from build123d import *

# Parameters (mm, degrees)
SKETCH_1_W           = 600
SKETCH_1_H           = 100
EXTRUDE_1_DEPTH      = 20
SKETCH_2_W           = 20
SKETCH_2_H           = 100
EXTRUDE_2_DEPTH      = 74
EXTRUDE_3_DEPTH      = 300
EXTRUDE_3_DEPTH_BACK = 300
SKETCH_3_W           = 20
SKETCH_3_H           = 20


with BuildPart() as part:
    # Эскиз1 → Выдавливание1 (new body)
    with BuildSketch(Plane(origin=(0, 0, 0), x_dir=(-1, 0, 0), z_dir=(0, 1, 0))):
        Rectangle(SKETCH_1_W, SKETCH_1_H)
    extrude(amount=EXTRUDE_1_DEPTH)

    # Эскиз2 → Выдавливание2 (add)
    with BuildSketch(Plane(origin=(0, 20, 0), x_dir=(-1, 0, 0), z_dir=(0, 1, 0))):
        with Locations((-290, 0)):
            Rectangle(SKETCH_2_W, SKETCH_2_H)
        with Locations((290, 0)):
            Rectangle(SKETCH_2_W, SKETCH_2_H)
    extrude(amount=EXTRUDE_2_DEPTH)

    # Эскиз3 → Выдавливание3 (add, two sides: drawn at the far end of the back side and taken through both)
    with BuildSketch(Plane.YZ.offset(-EXTRUDE_3_DEPTH_BACK)):
        with Locations((84, 60)):
            Rectangle(SKETCH_3_W, SKETCH_3_H)
    extrude(amount=EXTRUDE_3_DEPTH + EXTRUDE_3_DEPTH_BACK)


solid = part.part
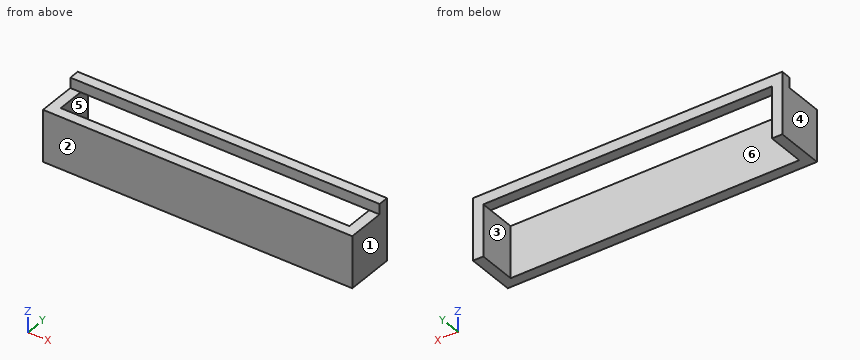
For this review, take the finished solid that the model builds, in its own axes (mm). Face numbers are marked on the shaded views. A direction names the side the tool comes from. Round coordinates to 2 decimals unless told otherwise and drop trailing zeros. Loops run counter-clockwise (first coordinate to the right, second up) from the corner with the lowest first, then second, coordinate; pieces in that order, holes last. Notation, with made-up numbers: (72, 58.25) - (87, 58.25) arc R30 ccw to (87, 82.25) - close; hole circle Ø8 at (6.5, -25). An arc over 180 degrees is marked (long way). Put each result on its own line as item: value. Start each with the question number.
1. Consider section A-A on y = 29. State the section outline as (x, z) points.
2. Consider section D-D on z = 59. State the section outline as (x, y) points, plus the area to 3 significant figures.
3. For the marked faces 4, 5 and 6, list the 3-axis set-ups (+Z, -Z, +X, -X, +Y, -Y) from which the entire face can be reached by the end or side of a thin tool; tool diameter is ignored.
4. Insertion check: P1, Ø6, axis at x = 122, y = 83.5, coming from the -Z side; P2, Ø6, axis at x = 23, z = 64, coming from the -Y side; P3, Ø1.5, axis at x = 66, y = 73.5, coming from the +Z side. Each pin has a flat end and moves straight along its axis. Give the tip position at first contact, or say it passes through.
5. For probe 1 along X at (y, z) = (65.5, -39); probe 2 along Y at (x, z) = (-206.5, -28.5); probe 3 along Z at (x, y) = (-123, 82.5), list the stretches that pass through material, from the lowest coordinate up. Write a range as [from, to].
6. Mouldability with a two-part tool opening along X and no side actions: class the marked faces 1, 2 and 3 as +X half, -X half, draft (parallel to the pull), parting line (faces both ways), or undercut.
7. Consider section C-C on z = 27.5. State the section outline as (x, y) points.
8. Consider section B-B on x = 96.5. State the section outline as (y, z) points, plus the area to 3 significant figures.
Result sheet:
1. outline: (-300, -50) - (-280, -50) - (-280, 50) - (-300, 50) - close; (280, -50) - (300, -50) - (300, 50) - (280, 50) - close
2. outline: (-300, 74) - (300, 74) - (300, 94) - (-300, 94) - close
2. area: 12,000 mm^2
3. face 4: +Z, -Z, -X, +Y, -Y
3. face 5: -Z, +Y
3. face 6: +Z, -Z, +Y
4. P1: z = 50
4. P2: y = 74
4. P3: z = 70
5. probe 1: [-300, -280], [280, 300]
5. probe 2: [0, 20]
5. probe 3: [50, 70]
6. face 1: +X half
6. face 2: draft
6. face 3: undercut
7. outline: (-300, 0) - (300, 0) - (300, 94) - (280, 94) - (280, 20) - (-280, 20) - (-280, 94) - (-300, 94) - close
8. outline: (0, -50) - (20, -50) - (20, 50) - (0, 50) - close; (74, 50) - (94, 50) - (94, 70) - (74, 70) - close
8. area: 2,400 mm^2
